Autodesk Inventor part; units mm, degrees
ref_plane "Work Plane1" through (0, 1, 0) normal (0, 1, 0) x (-1, 0, 0)
ref_plane "YZ Plane" through (0, 0, 0) normal (1, 0, 0) x (0, 1, 0)
ref_plane "XY Plane" through (0, 0, 0) normal (0, 0, 1) x (1, 0, 0)
sketch "Sketch1" plane through (0, 0, 0) normal (0, 1, 0) x (-1, 0, 0)
  circle A0 centre (0, 0) radius 12.5
  dimension "d0" = 25
extrude "Extrusion1" add sketch "Sketch1" along normal blind 4.5
ref_plane "Work Plane1" through (0, 1, 0) normal (0, 1, 0) x (-1, 0, 0)
sketch "Sketch2" plane through (0, 1, 0) normal (0, 1, 0) x (-1, 0, 0)
  line L0 (15, -1) -> (-15, -1)
  arc A0 (21, -27) -> (15, -1) centre (-24.8954, -23.8989) ccw
  line L1 (21, -27) -> (-21, -27)
  arc A1 (-15, -1) -> (-21, -27) centre (24.8954, -23.8989) ccw
  line L2 (-19.6045, -25.5298) -> (19.6045, -25.5298)
  arc A2 (19.6045, -25.5298) -> (14.1394, -2.4702) centre (-24.8954, -23.8989) ccw
  line L3 (14.1394, -2.4702) -> (-14.1394, -2.4702)
  arc A3 (-14.1394, -2.4702) -> (-19.6045, -25.5298) centre (24.8954, -23.8989) ccw
  point P0 (0, -1)
  point P1 (0, -27)
  dimension "d5" = 30
  dimension "d6" = 26
  dimension "d7" = 42
  dimension "d8" = 46
  dimension "d9" = 46
extrude "Extrusion2" add sketch "Sketch2" along normal blind 2.65
fillet "Fillet1" radius 2 1 edges at (12.5, 4.5, 0)
sketch "Sketch3" plane through (0, 0, 0) normal (0, -1, 0) x (1, 0, 0)
  line L0 (-7.886, 0) -> (-6.3799, 4.6353)
  line L1 (-6.3799, 4.6353) -> (-2.4369, 7.5)
  line L2 (-2.4369, 7.5) -> (2.4369, 7.5)
  line L3 (2.4369, 7.5) -> (6.3799, 4.6353)
  line L4 (6.3799, 4.6353) -> (7.886, 0)
  line L5 (7.886, 0) -> (6.3799, -4.6353)
  line L6 (6.3799, -4.6353) -> (2.4369, -7.5)
  line L7 (2.4369, -7.5) -> (-2.4369, -7.5)
  line L8 (-2.4369, -7.5) -> (-6.3799, -4.6353)
  line L9 (-6.3799, -4.6353) -> (-7.886, 0)
  point P0 (0, 0)
  point P1 (0, 0)
  point P2 (0, -7.5)
  dimension "d13" = 15
extrude "Extrusion3" add sketch "Sketch3" along normal blind 3
properties part number "brace_tabs_half"
The model under review builds one solid part; all positions refer to its coordinate system, in mm. A direction names the side the tool comes from. Round coordinates to 2 decimals unless told otherwise and drop trailing zeros. Write each loop counter-clockwise with the first axis right and the second up, starting at its lowest first coordinate (ties: lowest second). Pieces come first, ordered by that corner, then holes. Notation, with made-up numbers: (4, 7.25) - (43, 7.25) arc R10 cw to (43, 14.25) - close; hole circle Ø1 at (57, 67). An arc over 180 degrees is marked (long way). Answer as CSV lines item,"result". Start each with the question number.
(1) For pin 1 Ø8 at (x, z) = (-6, -10) entering from -Y; pin 2 Ø2.5 at (x, y) = (-0.5, -1) entering from -Z; pin 3 Ø3 at (x, y) = (6.5, 2.5) entering from +Z; pin 4 Ø3 at (x, z) = (6.5, -12.5) entering from -Y, all flat-tipped, find the tip position at first contact; note any pin that passes through.
(2) Draft analysis for pull direction Z (two halves, no side actions). For faces 4 (the flat face through (7.14, -1.48, -2.29)), 5 (the flat face through (-4.436, -1.479, 6.048)), 6 (the flat face through (0, 2, -25.53)), 7 (the cylindrical face through (-11.923, 1.232, -3.755)), state which applies: pulls with the +Z half, pulls with the -Z half, needs draft (parallel to the pull), parting line crosses it, or undercut.
(3) We need section A-A on x = -13.5. State the section outline as (y, z) points, plus the area to 3 significant figures.
(4) We need section C-C on x = 0. State the section outline as (y, z) points.
(5) We need section B-B on z = -17. State the section outline as (x, y) points.
(6) To check wall thickness, follow line 1 (X direction, y = 3, z = -6); line 2 (Z direction, x = 14, y = 3.25); line 3 (X direction, y = 2.75, z = -6.5). State the ranges of each line that lie inside material, in increasing order.
(7) For faces 1 (the flat face through (0, -1, 7.5)), 2 (the flat face through (-7.122, -1.479, -2.35)), 3 (the flat face through (0, 0, -8)), list the 3-axis set-ups (+Z, -Z, +X, -X, +Y, -Y) from which the entire face can be reached by the end or side of a thin tool; tool diameter is ignored.
Worked answers:
1,pin 1,"y = 0"
1,pin 2,"z = -12.5"
1,pin 3,"z = 11.46"
1,pin 4,"through"
2,face 4,"pulls with the -Z half"
2,face 5,"pulls with the +Z half"
2,face 6,"undercut"
2,face 7,"undercut"
3,outline,"(1, -27) - (3.65, -27) - (3.65, -25.53) - (1, -25.53) - close; (1, -2.47) - (3.65, -2.47) - (3.65, -1) - (1, -1) - close"
3,area,"7.79 mm²"
4,outline,"(-3, -7.5) - (0, -7.5) - (0, -12.5) - (2.5, -12.5) arc R2 ccw to (4.5, -10.5) - (4.5, 10.5) arc R2 ccw to (2.5, 12.5) - (0, 12.5) - (0, 7.5) - (-3, 7.5) - close; (1, -27) - (3.65, -27) - (3.65, -25.53) - (1, -25.53) - close"
5,outline,"(-20.58, 1) - (-19.1, 1) - (-19.1, 3.65) - (-20.58, 3.65) - close; (19.1, 1) - (20.58, 1) - (20.58, 3.65) - (19.1, 3.65) - close"
6,line 1,"-17.48 to -15.88, -10.89 to 10.89, 15.88 to 17.48"
6,line 2,"-27 to -25.53, -2.47 to -1"
6,line 3,"-17.69 to -16.09, -10.66 to 10.66, 16.09 to 17.69"
7,face 1,"+Z, +X, -X, -Y"
7,face 2,"-Z, -X, -Y"
7,face 3,"-Y"
